```python
from build123d import *

# Parameters (mm, degrees)
BOSS_EXTRUDE1_DEPTH = 282
BOSS_EXTRUDE2_DEPTH = 62


with BuildPart() as part:
    # Sketch1 → Boss-Extrude1 (new body)
    with BuildSketch(Plane.XY):
        Polygon((-2.36, 23.687204572), (59.64, 23.687204572), (59.64, 16.298774949), (62.34, 16.298774949), (62.34, 10.337204572), (59.54, 10.337204572), (59.54, 13.512204572), (56.94, 13.512204572), (56.94, 20.512204572), (0.34, 20.512204572), (0.34, 13.512204572), (-2.26, 13.512204572), (-2.26, 10.337204572), (-5.06, 10.337204572), (-5.06, 16.298774949), (-2.36, 16.298774949), align=None)
    extrude(amount=BOSS_EXTRUDE1_DEPTH)

    # Sketch5 → Boss-Extrude2 (add)
    with BuildSketch(Plane.ZY.offset(2.36)):
        Polygon((0, 23.687204572), (-5.1, 23.687204572), (-5.1, 19.473774949), (-14.890029998, 19.473774949), (-14.890029998, 10.337204572), (-11.715029998, 10.337204572), (-11.715029998, 16.298774949), (-1.925, 16.298774949), (-1.925, 20.512204572), (0, 20.512204572), align=None)
    extrude(amount=-BOSS_EXTRUDE2_DEPTH)


solid = part.part
```
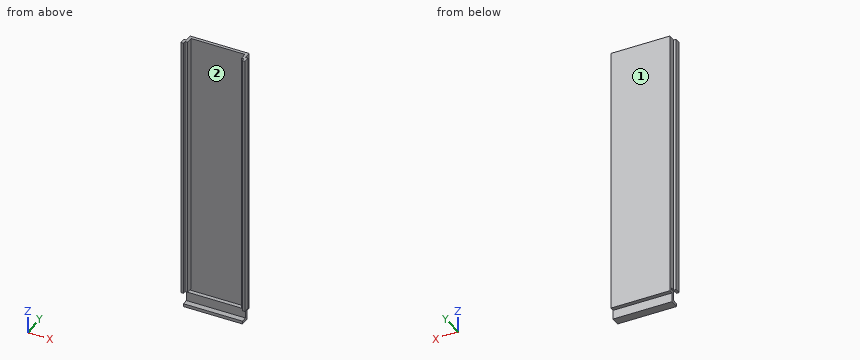
Part model, mm, in its own coordinate system. Face numbers are marked on the shaded views. Coordinates: 2 decimals unless noted, no trailing zeros. Loops run counter-clockwise (first coordinate to the right, second up) from the corner with the lowest first, then second, coordinate; pieces in that order, holes last. Notation, with made-up numbers: (-18.5, 49) - (12.5, 49) arc R7 ccw to (12.5, 61) - close; hole circle Ø10 at (-24.5, 58.5). An arc over 180 degrees is marked (long way). Write item = value, one per line. Start each with the question number.
Item 1: Cut at B-B, the plane x = 15.5. Give the cut face in (y, z) (3 decimals), and give its area (3 significant figures).
Item 2: Flat gauge pins, fed straight in: pin 1 Ø3 at (x, z) = (28.5, -7) entering from -Y; pin 2 Ø1 at (x, z) = (9.5, 80) entering from -Y; pin 3 Ø1 at (y, z) = (17.5, 122.5) entering from -X. Where does each tip first touch, or does it go through?
Item 3: Wall check: L1, parallel to X at y = 14.5, z = 191; L2, parallel to X at y = 11.75, z = 253.5; L3, parallel to Z at x = -1.5, y = 14.5. Give the ranges that are in metal, low to high. Write a range as from..to.
Item 4: Mould opens along X. For the marked faces 1 and 2 say: released by +X, released by -X, zero draft, split by the parting line, or undercut.
Item 5: Cut at A-A, the plane z = 191. Give the cut face in (x, y).
The answers:
q1.outline = (10.337, -14.89) - (19.474, -14.89) - (19.474, -5.1) - (23.687, -5.1) - (23.687, 282) - (20.512, 282) - (20.512, -1.925) - (16.299, -1.925) - (16.299, -11.715) - (10.337, -11.715) - close
q1.area = 975 mm2
q2.pin_1 = 16.3
q2.pin_2 = 20.51
q2.pin_3 = -2.36
q3.L1 = -5.06..0.34, 56.94..62.34
q3.L2 = -5.06..-2.26, 59.54..62.34
q3.L3 = -14.89..-11.72, 0..282
q4.face_1 = zero draft
q4.face_2 = undercut
q5.outline = (-5.06, 10.34) - (-2.26, 10.34) - (-2.26, 13.51) - (0.34, 13.51) - (0.34, 20.51) - (56.94, 20.51) - (56.94, 13.51) - (59.54, 13.51) - (59.54, 10.34) - (62.34, 10.34) - (62.34, 16.3) - (59.64, 16.3) - (59.64, 23.69) - (-2.36, 23.69) - (-2.36, 16.3) - (-5.06, 16.3) - close
